The figure shows three views and two pictorial views of one solid part (mm, origin at its lowest corner). Answer the questions. Round coordinates to 2 decimals unless told otherwise and drop trailing zeros. Order: outer loops, then holes, each group sorted by start corner. A loop starts at its lowest first (then second) coordinate and runs counter-clockwise, first axis right, second up. Notation, with made-up numbers: M 20.5,69.25 L 59.5,69.25 A18 ccw 59.5,73.25 Z; hole C 22,30 d5. An arc over 180 degrees is marked long. Answer as CSV lines item,"result".
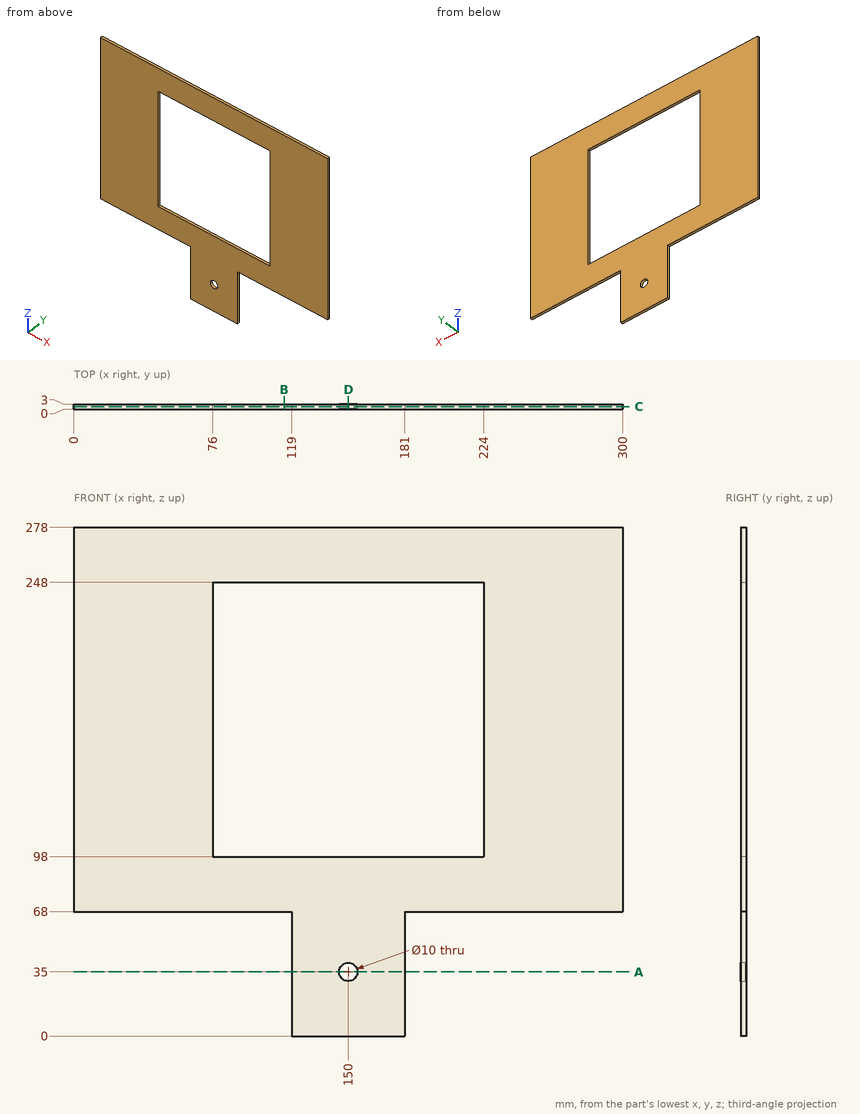
Item 1: A cutting plane is placed at B-B, the plane x = 115. Determine the outline of the cut face in (y, z).
Ans:
outline,"M 0,68 L 3,68 L 3,98 L 0,98 Z; M 0,248 L 3,248 L 3,278 L 0,278 Z"
Item 2: A cutting plane is placed at C-C, the plane y = 1.5. Determine the outline of the cut face in (x, z).
Ans:
outline,"M 0,68 L 119,68 L 119,0 L 181,0 L 181,68 L 300,68 L 300,278 L 0,278 Z; hole M 76,98 L 224,98 L 224,248 L 76,248 Z; hole C 150,35 d10"
Item 3: A cutting plane is placed at D-D, the plane x = 150. Determine the outline of the cut face in (y, z), and give its area (3 significant figures).
Ans:
outline,"M 0,0 L 3,0 L 3,30 L 0,30 Z; M 0,40 L 3,40 L 3,98 L 0,98 Z; M 0,248 L 3,248 L 3,278 L 0,278 Z"
area,"354 mm2"
Item 4: Flat-ended cylindrical pins translate along their axes: pin 1 (1 mm diameter, centred on x = 32, y = 1.5, fed in from -Z); pin 2 (10 mm diameter, centred on x = 56, z = 61.5, fed in from -Y); pin 3 (0.9 mm diameter, centred on y = 1.5, z = 38, fed in from -X). Find the tip coordinate at first contact, or state that the pin passes through.
Ans:
pin 1,"z = 68"
pin 2,"through"
pin 3,"x = 119"
Item 5: Find the intervals of material crossed by probe 1 along X at (y, z) = (1.6, 201); probe 2 along Z at (x, y) = (98.5, 2.5); probe 3 along Z at (x, y) = (165, 1.5), in increasing order. Write a range as [from, to].
Ans:
probe 1,"[0, 76], [224, 300]"
probe 2,"[68, 98], [248, 278]"
probe 3,"[0, 98], [248, 278]"
Item 6: A cutting plane is placed at A-A, the plane z = 35. Determine the outline of the cut face in (x, y), and give its area (3 significant figures).
Ans:
outline,"M 119,0 L 145,0 L 145,3 L 119,3 Z; M 155,0 L 181,0 L 181,3 L 155,3 Z"
area,"156 mm2"
